Source: CAD feature listing. Evaluate the final solid. Frame: model axes, mm. Face numbers are marked on the shaded views. A direction names the side the tool comes from. Round coordinates to 2 decimals unless told otherwise and drop trailing zeros. Order: outer loops, then holes, each group sorted by start corner. A loop starts at its lowest first (then second) coordinate and runs counter-clockwise, first axis right, second up. Notation, with made-up numbers: (79.5, 62) -> (115.5, 62) arc R8 ccw to (115.5, 76) -> close; hole circle Ø6 at (-20, -14.5). An arc over 180 degrees is marked (long way). Answer as CSV lines item,"result". Start each with the question number.
(1) Pull-direction query (Z, two-part tool) for the marked faces 1, 2 and 3; classes: +Z half, -Z half, draft (parallel to the pull), parting line (faces both ways), or undercut.
(2) Section query C-C (z = -5.5). Output: boundary loops of the cut face in (x, y), plus the area to 3 significant figures.
(3) Contact query for flat-ended pins moving along their axis: P1, Ø4, axis at y = 3, z = -3.5, coming from the -X side; P2, Ø5.5, axis at y = 9, z = 0.5, coming from the +X side; P3, Ø7, axis at x = 0, y = 0, coming from the -Z side; P4, Ø8, axis at x = 16.5, z = -2.5, coming from the +Y side. Output: stop coordinate, or through.
(4) Section query A-A (y = 10.5). Output: boundary loops of the cut face in (x, z), plus the area to 3 significant figures.
(5) Line query: line 1 along X through (y, z) = (-20.2, 0); line 2 along Y through (x, z) = (-7.75, 0); line 3 along X through (y, z) = (-18, 0.75). Output: solid intervals per line, ascending. Write a range as from..to.
(6) Section query D-D (x = 4.5). Count the separate pieces of the cut face and the enclosed holes in it, plus the area to 3 significant figures.
(7) Section query B-B (y = 0). Output: boundary loops of the cut face in (x, z), plus the area to 4 significant figures.
(8) Set-up query: the marked faces 4, 5 and 6. Return all of +Z, -Z, +X, -X, +Y, -Y with unobstructed straight access to the full face (end or side cutting, diameter ignored); none if empty.
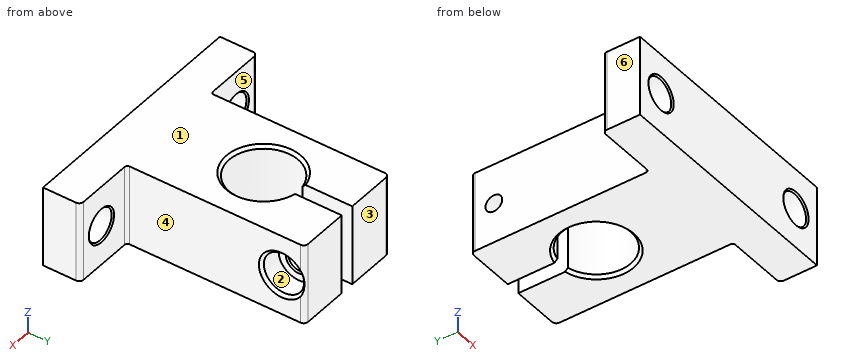
```python
from build123d import *

# Parameters (mm, degrees)
BOSS_EXTRUDE1_DEPTH                 = 7
F_5_5_5_5_DIAMETER_HOLE2_AT_2_COUNT = 2
F_5_5_5_5_DIAMETER_HOLE2_AT_2_PITCH = 32
M3_5X0_6_TAPPED_HOLE1_D             = 2.9
M3_5X0_6_TAPPED_HOLE1_DEPTH         = 8.75
FILLET1_R                           = 0.75
FILLET1_2_R                         = 0.5
CHAMFER1_SIZE                       = 0.5


with BuildPart() as part:
    # Sketch2 → Boss-Extrude1 (new body, symmetric)
    with BuildSketch(Plane.XY):
        with BuildLine():
            Line((-21, -16.5), (-10, -16.5))
            Line((-10, -16.5), (-10, 14.5))
            Line((-10, 14.5), (-1.25, 14.5))
            Line((-1.25, 14.5), (-1.25, 5.868347297))
            ThreePointArc((-1.25, 5.868347297), (0, -6), (1.25, 5.868347297))
            Line((1.25, 5.868347297), (1.25, 14.5))
            Line((1.25, 14.5), (10, 14.5))
            Line((10, 14.5), (10, -16.5))
            Line((10, -16.5), (21, -16.5))
            Line((21, -16.5), (21, -23))
            Line((21, -23), (-21, -23))
            Line((-21, -23), (-21, -16.5))
        make_face()
    extrude(amount=BOSS_EXTRUDE1_DEPTH, both=True)

    # Sketch5 → 5.5 _5.5_ Diameter Hole2 (revolve, cut)
    with BuildSketch(Plane(origin=(-16, -16.5, 0), x_dir=(0, 0, 1), z_dir=(1, 0, 0))):
        Polygon((0, 0), (0, 6.5), (3, 6.5), (2.75, 6.25), (2.75, 0.25), (3, 0), align=None)
    f_5_5_5_5_diameter_hole2 = revolve(axis=Axis((-16, -10.15, 0), (0, -1, 0)), mode=Mode.SUBTRACT)

    # 5.5 _5.5_ Diameter Hole2 at 2: 5.5 _5.5_ Diameter Hole2 ×2
    with Locations(*[(i * F_5_5_5_5_DIAMETER_HOLE2_AT_2_PITCH, 0, 0) for i in range(1, F_5_5_5_5_DIAMETER_HOLE2_AT_2_COUNT)]):
        add(f_5_5_5_5_diameter_hole2, mode=Mode.SUBTRACT)

    # M3.5x0.6 Tapped Hole1
    with Locations(Plane.ZY.offset(10)):
        with Locations((0, 10.5)):
            Hole(M3_5X0_6_TAPPED_HOLE1_D / 2, depth=M3_5X0_6_TAPPED_HOLE1_DEPTH)

    # Fillet1
    fillet1_edges = [part.edges().sort_by_distance(p)[0] for p in [
        (10, 14.5, 0),
        (-10, 14.5, 0),
        (21, -16.5, 0),
        (-21, -16.5, 0),
    ]]
    fillet(fillet1_edges, radius=FILLET1_R)

    # Fillet1 2
    fillet1_2_edges = [part.edges().sort_by_distance(p)[0] for p in [
        (10, -16.5, 0),
        (-10, -16.5, 0),
    ]]
    fillet(fillet1_2_edges, radius=FILLET1_2_R)

    # Sketch12 → CBORE for M5 Hex Head Bolt1 (revolve, cut)
    with BuildSketch(Plane(origin=(10, 10.5, 0), x_dir=(0, 0, -1), z_dir=(0, 1, 0))):
        Polygon((0, 0), (0, 8.75), (2, 8.75), (2, 4.25), (2.25, 4), (3.5, 4), (3.5, 0.5), (4, 0), align=None)
    revolve(axis=Axis((16.35, 10.5, 0), (-1, 0, 0)), mode=Mode.SUBTRACT)

    # Chamfer1
    chamfer1_edges = [part.edges().sort_by_distance(p)[0] for p in [
        (0, -6, 7),
        (0, -6, -7),
    ]]
    chamfer(chamfer1_edges, length=CHAMFER1_SIZE)


solid = part.part
```
Answer block:
1,face 1,"+Z half"
1,face 2,"undercut"
1,face 3,"draft"
2,outline,"(-21, -23) -> (21, -23) -> (21, -17.25) arc R0.75 ccw to (20.25, -16.5) -> (10.5, -16.5) arc R0.5 cw to (10, -16) -> (10, 13.75) arc R0.75 ccw to (9.25, 14.5) -> (1.25, 14.5) -> (1.25, 5.87) arc R6 cw (long way) to (-1.25, 5.87) -> (-1.25, 14.5) -> (-9.25, 14.5) arc R0.75 ccw to (-10, 13.75) -> (-10, -16) arc R0.5 cw to (-10.5, -16.5) -> (-20.25, -16.5) arc R0.75 ccw to (-21, -17.25) -> close"
2,area,"758 mm2"
3,P1,"x = -10"
3,P2,"x = 10"
3,P3,"through"
3,P4,"y = -16.5"
4,outline,"(-10, -7) -> (-1.25, -7) -> (-1.25, -1.45) -> (-10, -1.45) -> close; (-10, 1.45) -> (-1.25, 1.45) -> (-1.25, 7) -> (-10, 7) -> close; (1.25, -7) -> (10, -7) -> (10, -4) -> (9.5, -3.5) -> (6, -3.5) -> (6, -2.25) -> (5.75, -2) -> (1.25, -2) -> close; (1.25, 2) -> (5.75, 2) -> (6, 2.25) -> (6, 3.5) -> (9.5, 3.5) -> (10, 4) -> (10, 7) -> (1.25, 7) -> close"
4,area,"172 mm2"
5,line 1,"-21..-18.75, -13.25..13.25, 18.75..21"
5,line 2,"-23..9.05, 11.95..14.5"
5,line 3,"-21..-18.65, -13.35..13.35, 18.65..21"
6,separate pieces,"2"
6,enclosed holes,"1"
6,area,"401 mm2"
7,outline,"(-10, -7) -> (-6.5, -7) -> (-6, -6.5) -> (-6, 6.5) -> (-6.5, 7) -> (-10, 7) -> close; (6, -6.5) -> (6.5, -7) -> (10, -7) -> (10, 7) -> (6.5, 7) -> (6, 6.5) -> close"
7,area,"111.5 mm2"
8,face 4,"+Z, -Z, +X, +Y"
8,face 5,"+Z, -Z, -X, +Y"
8,face 6,"+Z, -Z, -X, +Y, -Y"
